Can you work these out from the model? Positions are in its coordinate system, mm. A direction names the side the tool comes from. Round coordinates to 2 decimals unless told otherwise and drop trailing zeros. Write each loop counter-clockwise with the first axis right and the second up, starting at its lowest first coordinate (ties: lowest second). Pieces come first, ordered by that corner, then holes. Notation, with made-up numbers: (57.5, 81.5) -> (101.5, 81.5) arc R22 ccw to (101.5, 118.5) -> close; hole circle Ø11 at (62, 84). An arc over 180 degrees is marked (long way). Write item = value, one per line. Start each with the question number.
1) Imagine slicing it at A-A, the plane x = 0. Please give me the cut outline in (y, z) (3 decimals).
2) For faces 1 (the face through (-0.59, 4.46, 3.45)), 2 (the face through (-0.465, 3.545, 2.566)), which set-ups out of +Z, -Z, +X, -X, +Y, -Y let a thin tool reach every point of the face, with its end or its side?
3) Imagine slicing it at C-C, the plane z = 6. Please give me the cut outline in (x, y), then the cut area to 3 significant figures.
4) Imagine slicing it at D-D, the plane z = 3.75. Please give me the cut outline in (x, y) (3 decimals).
5) I'm going to push flat-ended pins straight in: pin 1 (1.5 mm diameter, centred on y = 1, z = 1.5, fed in from -X); pin 2 (1 mm diameter, centred on x = 1.5, z = 1.5, fed in from +Y); pin 3 (1 mm diameter, centred on y = 2, z = 3, fed in from +X). Where does each tip first touch, or does it pass through?
6) If I drill on line 1 (Y direction, x = 0, z = 5.4); line 2 (Y direction, x = 0, z = 3.35) (3 decimals); line 3 (Z direction, x = -2, y = 2), over which ranges is the centre line in solid material (lowest first)?
from build123d import *

# Parameters (mm, degrees)
F0_R     = 4.5
F0_R_2   = 3.575
F1_DEPTH = 5
F4_R     = 4.5
F4_R_2   = 2
F5_DEPTH = 2
F6_R     = 0.2


with BuildPart() as f1:
    # F0 (on Top) → F1 (new body)
    with BuildSketch(Plane.XY):
        Circle(F0_R)
        Circle(F0_R_2, mode=Mode.SUBTRACT)
    extrude(amount=F1_DEPTH)

    # F2 (on Front) → F3 (revolve, cut)
    with BuildSketch(Plane.XZ):
        with BuildLine():
            Line((0, 12), (0, 22))
            ThreePointArc((0, 22), (-5, 17), (0, 12))
        make_face()
    revolve(axis=Axis((0, 0, 14.014009), (0, 0, 1)), mode=Mode.SUBTRACT)

    # F4 (on face) → F5 (join)
    with BuildSketch(Plane.XY.offset(5)):
        Circle(F4_R)
        Circle(F4_R_2, mode=Mode.SUBTRACT)
    extrude(amount=F5_DEPTH)

    # F6
    f6_edges = [f1.edges().sort_by_distance(p)[0] for p in [
        (-4.5, 0, 0),
        (4.5, 0, 3.5),
        (-4.5, 0, 7),
        (-2, 0, 7),
        (-3.575, 0, 0),
    ]]
    fillet(f6_edges, radius=F6_R)


solid = f1.part
Reported:
q1.outline = (-4.5, 0.2) arc R0.2 ccw to (-4.3, 0) -> (-3.775, 0) arc R0.2 ccw to (-3.575, 0.2) -> (-3.575, 5) -> (-2, 5) -> (-2, 6.8) arc R0.2 ccw to (-2.2, 7) -> (-4.3, 7) arc R0.2 ccw to (-4.5, 6.8) -> close; (2, 5) -> (3.575, 5) -> (3.575, 0.2) arc R0.2 ccw to (3.775, 0) -> (4.3, 0) arc R0.2 ccw to (4.5, 0.2) -> (4.5, 6.8) arc R0.2 ccw to (4.3, 7) -> (2.2, 7) arc R0.2 ccw to (2, 6.8) -> close
q2.face_1 = +Z, -Z
q2.face_2 = -Z
q3.outline = circle Ø9 at (0, 0); hole circle Ø4 at (0, 0)
q3.area = 51.1 mm²
q4.outline = circle Ø9 at (0, 0); hole circle Ø7.15 at (0, 0)
q5.pin_1 = -4.49
q5.pin_2 = 4.39
q5.pin_3 = 4.24
q6.line_1 = -4.5 to -2, 2 to 4.5
q6.line_2 = -4.5 to -3.575, 3.575 to 4.5
q6.line_3 = 5 to 7
